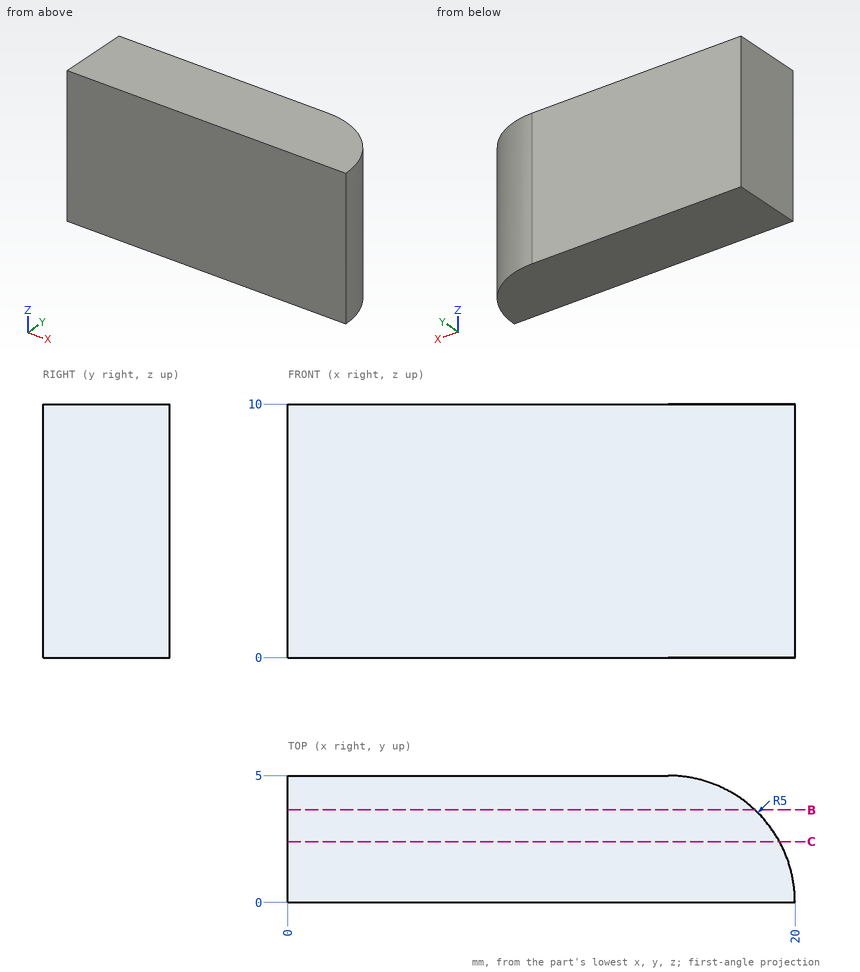
Job drawing, mm, ordinate dimensions from the low corner. One solid piece. Give positions to 0.01 mm unless a question says otherwise; leave off trailing zeros. Order: outer loops, then holes, each group sorted by start corner. A loop starts at its lowest first (then second) coordinate and runs counter-clockwise, first axis right, second up. Notation, with made-up numbers: (71.5, 44) - (109.5, 44) arc R22 cw to (109.5, 81) - close; hole circle Ø5 at (11.5, 78). An arc over 180 degrees is marked (long way). Return JSON: item names as keys, results as strings.
1) Probe line 1 (X direction, y = 0.35, z = 7); line 2 (X direction, y = 3.7, z = 5.5); line 3 (Y direction, x = 18, z = 5.25). List the from-to ranges inside material, lowest first. Write a range as from..to.
Geometry says:
{"line 1": "0..19.99", "line 2": "0..18.36", "line 3": "0..4"}
2) Cut at B-B, the plane y = 3.65. Give the cut face in (x, z).
Geometry says:
{"outline": "(0, 0) - (18.42, 0) - (18.42, 10) - (0, 10) - close"}
3) Cut at C-C, the plane y = 2.4. Give the cut face in (x, z).
Geometry says:
{"outline": "(0, 0) - (19.39, 0) - (19.39, 10) - (0, 10) - close"}
4) Flat gauge pin, fed straight in: P1, Ø1.5, axis at y = 4, z = 8, coming from the +X side. Where does the tip first touch, or does it go through?
Geometry says:
{"P1": "x = 18.8"}
